from build123d import *

# Parameters (mm, degrees)
P_IDAT_VYSUNUT_M1_DEPTH = 3
P_IDAT_VYSUNUT_M2_DEPTH = 2
ZAOBLIT1_R              = 1


with BuildPart() as part:
    # Skica1 → P_idat vysunut_m1 (new body)
    with BuildSketch(Plane(origin=(0, 0, 0), x_dir=(1, 0, 0), z_dir=(0, 1, 0))):
        Polygon((26.667853432, 46.190077074), (13.677472376, 53.690077074), (11.737150801, 42.685966604), (0.392218012, 49.235966604), (10.61747027, 66.946623035), (-0.554257439, 73.396623035), (-2.393036353, 62.968389614), (-13.22114317, 69.22), (-52.538696502, 46.52), (-91.856249834, 69.22), (-91.856249834, 37.22), (-73.49138407, 28.419769911), (-45.928124917, 0), (0, 0), align=None)
    extrude(amount=P_IDAT_VYSUNUT_M1_DEPTH)

    # Skica1_15 → P_idat vysunut_m2 (add)
    with BuildSketch(Plane(origin=(0, 0, 0), x_dir=(1, 0, 0), z_dir=(0, 1, 0))):
        Polygon((-91.856249834, 0), (-45.928124917, 0), (-73.49138407, 28.419769911), (-91.856249834, 37.22), (-91.856249834, 33.55662508), (-91.856249834, 24.27831254), (-81.356249834, 24.27831254), (-81.356249834, 11.17831254), (-91.856249834, 15), (-91.856249834, 1.897719633), align=None)
        Polygon((-91.856249834, 24.27831254), (-91.856249834, 33.55662508), (-101.80675435, 37.17831254), (-101.80675435, 24.27831254), align=None)
    extrude(amount=P_IDAT_VYSUNUT_M2_DEPTH)

    # Zaoblit1
    zaoblit1_edges = [part.edges().sort_by_distance(p)[0] for p in [
        (10.61747027, 1.5, -66.946623035),
        (0.392218012, 1.5, -49.235966604),
        (11.737150801, 1.5, -42.685966604),
        (13.677472376, 1.5, -53.690077074),
        (0, 1.5, 0),
        (-2.393036353, 1.5, -62.968389614),
        (-0.554257439, 1.5, -73.396623035),
        (-91.856249834, 1, -33.55662508),
        (-101.80675435, 1, -37.17831254),
        (-101.80675435, 1, -24.27831254),
        (-81.356249834, 1, -24.27831254),
        (-81.356249834, 1, -11.17831254),
        (-91.856249834, 1, -15),
    ]]
    fillet(zaoblit1_edges, radius=ZAOBLIT1_R)


solid = part.part
The model under review builds one solid part; all positions refer to its coordinate system, in mm. A direction names the side the tool comes from. Round coordinates to 2 decimals unless told otherwise and drop trailing zeros. Write each loop counter-clockwise with the first axis right and the second up, starting at its lowest first coordinate (ties: lowest second). Pieces come first, ordered by that corner, then holes. Notation, with made-up numbers: (53, 24.25) -> (93, 24.25) arc R28 cw to (93, 63.25) -> close; hole circle Ø4 at (7, -6.5). An arc over 180 degrees is marked (long way). Answer as a JSON object with one key per item and string values.
1. We need section D-D on z = -40. State the section outline as (x, y) points.
Results found:
{"outline": "(-91.86, 0) -> (23.09, 0) -> (23.09, 3) -> (-91.86, 3) -> close"}
2. We need section A-A on z = -58. State the section outline as (x, y) points.
Results found:
{"outline": "(-91.86, 0) -> (-72.42, 0) -> (-72.42, 3) -> (-91.86, 3) -> close; (-32.65, 0) -> (5.45, 0) -> (5.45, 3) -> (-32.65, 3) -> close"}
3. We need section B-B on y = 2.5. State the section outline as (x, z) points.
Results found:
{"outline": "(-91.86, -69.22) -> (-52.54, -46.52) -> (-13.22, -69.22) -> (-3.63, -63.68) arc R1 cw to (-2.15, -64.37) -> (-0.8, -71.99) arc R1 ccw to (0.68, -72.68) -> (9.75, -67.45) arc R1 ccw to (10.12, -66.08) -> (0.89, -50.1) arc R1 cw to (1.26, -48.74) -> (10.5, -43.4) arc R1 cw to (11.99, -44.09) -> (13.43, -52.28) arc R1 ccw to (14.91, -52.98) -> (26.67, -46.19) -> (0.29, -0.5) arc R1 ccw to (-0.58, 0) -> (-45.93, 0) -> (-73.49, -28.42) -> (-91.86, -37.22) -> close"}
4. Clearance check with flat-ended pins moving along their axes: pin 1 (1.5 mm diameter, centred on x = 1, y = 0.5, fed in from -Z); pin 2 (3 mm diameter, centred on x = -43.5, z = -11, fed in from -Y); pin 3 (0.9 mm diameter, centred on y = 1, z = -59, fed in from -X); pin 4 (1.5 mm diameter, centred on x = 4.5, y = 1.5, fed in from +Z). State where each tip first meets the part, or that it passes through.
Results found:
{"pin 1": "stops at z = -72.81", "pin 2": "stops at y = 0", "pin 3": "stops at x = -91.86", "pin 4": "stops at z = -6.5"}
5. Machinability: for faces 5 (the face through (-86.55, 0.99, -13.07)), 6 (the face through (-1.464, 1.479, -68.236)), 7 (the face through (-47, 1, 0)), 8 (the face through (-74, 2, -15)), 9 (the face through (20.873, 1.479, -49.536)), which of the approach directions +Z, -Z, +X, -X, +Y, -Y give a long, thin tool a straight path to every point of the face, cutting with its end or side? Answer none if there is none.
Results found:
{"face 5": "+Y, -Y", "face 6": "-Z, +Y, -Y", "face 7": "+Z, +X, -X, +Y, -Y", "face 8": "+Z, -X, +Y", "face 9": "-Z, +X, +Y, -Y"}
6. We need section C-C on x = -48. State the section outline as (y, z) points.
Results found:
{"outline": "(0, -49.14) -> (3, -49.14) -> (3, -2.14) -> (2, -2.14) -> (2, 0) -> (0, 0) -> close"}
7. The part is to be moulded in two halves that separate along Z. For faces 1 (the face through (-33, 3, -37)), 2 (the face through (5.44, 1.48, -57.98)), 3 (the face through (6, 1, -46)), 4 (the face through (-96.78, 0.99, -35.35)), say which applies: pulls with the +Z half, pulls with the -Z half, needs draft (parallel to the pull), parting line crosses it, or undercut.
Results found:
{"face 1": "needs draft", "face 2": "undercut", "face 3": "undercut", "face 4": "pulls with the -Z half"}
8. To check wall thickness, follow line 1 along X through (y, z) = (0.4, -65.5); line 2 along X through (y, z) = (1.6, -66); line 3 along Z through (x, y) = (1.5, 2.5). State the ranges of each line that lie inside material, in increasing order.
Results found:
{"line 1": "x = -91.86 to -85.41, -19.66 to -6.78, -1.95 to 9.78", "line 2": "x = -91.86 to -86.28, -18.8 to -7.64, -1.86 to 10.07", "line 3": "z = -72.21 to -51.15, -48.6 to -2.6"}
